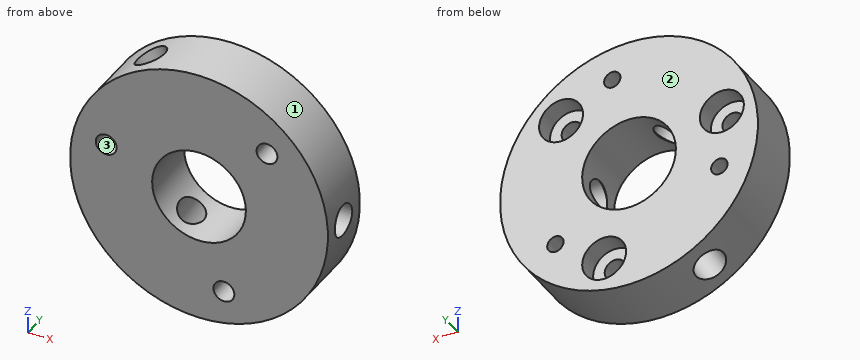
```python
from build123d import *

# Parameters (mm, degrees)
SKETCH1_R                                      = 13.97
BOSS_EXTRUDE1_DEPTH                            = 6.35
CBORE_FOR_2_SOCKET_HEAD_CAP_SCREW1_D           = 2.2606
CBORE_FOR_2_SOCKET_HEAD_CAP_SCREW1_CBORE_D     = 4.7625
CBORE_FOR_2_SOCKET_HEAD_CAP_SCREW1_CBORE_DEPTH = 2.1844
CIRPATTERN1_COUNT                              = 3
CIRPATTERN2_COUNT                              = 3
CIRPATTERN3_COUNT                              = 3
CUT_EXTRUDE2_REACH                             = 22.752
SKETCH16_R                                     = 5.08


with BuildPart() as part:
    # Sketch1 → Boss-Extrude1 (new body)
    with BuildSketch(Plane(origin=(0, 0, 0), x_dir=(1, 0, 0), z_dir=(0, 1, 0))):
        with Locations(Location((0, 0, 0), (0, 0, 270))):
            Circle(SKETCH1_R)
    extrude(amount=BOSS_EXTRUDE1_DEPTH)

    # CBORE for #2 Socket Head Cap Screw1 (through all)
    with Locations(Plane(origin=(0, 6.35, 0), x_dir=(1, 0, 0), z_dir=(0, 1, 0))):
        with Locations((7.363810019, -7.363810019)):
            cbore_for_2_socket_head_cap_screw1 = CounterBoreHole(CBORE_FOR_2_SOCKET_HEAD_CAP_SCREW1_D / 2, CBORE_FOR_2_SOCKET_HEAD_CAP_SCREW1_CBORE_D / 2, CBORE_FOR_2_SOCKET_HEAD_CAP_SCREW1_CBORE_DEPTH)

    # CirPattern1: CBORE for #2 Socket Head Cap Screw1 ×3 about axis
    cirpattern1_axis = Axis((0, 0, 0), (0, 1, 0))
    for i in range(1, CIRPATTERN1_COUNT):
        add(cbore_for_2_socket_head_cap_screw1.rotate(cirpattern1_axis, i * 360 / CIRPATTERN1_COUNT), mode=Mode.SUBTRACT)

    # Sketch10 → Tap Drill for #2-56 Tap2 (revolve, cut)
    with BuildSketch(Plane(origin=(7.977586831, 6.35, -6.693990167), x_dir=(0, 0, 1), z_dir=(1, 0, 0))):
        Polygon((0, 0), (0, 4.59816509), (0.889, 4.064), (0.889, 0), align=None)
    tap_drill_for_2_56_tap2 = revolve(axis=Axis((7.977586831, 12.7, -6.693990167), (0, -1, 0)), mode=Mode.SUBTRACT)

    # CirPattern2: Tap Drill for #2-56 Tap2 ×3 about axis
    cirpattern2_axis = Axis((0, 0, 0), (0, 1, 0))
    for i in range(1, CIRPATTERN2_COUNT):
        add(tap_drill_for_2_56_tap2.rotate(cirpattern2_axis, i * 360 / CIRPATTERN2_COUNT), mode=Mode.SUBTRACT)

    # Sketch15 → Tap Drill for #8-32 Tap2 (revolve, cut)
    with BuildSketch(Plane(origin=(-6.942501454, 3.105629072, 12.122812114), x_dir=(0.8677746681735182, 0, 0.4969578707258195), z_dir=(0, 1, 0))):
        Polygon((0, 0), (0, 10.339292883), (1.7272, 8.89), (1.7272, 0), align=None)
    tap_drill_for_8_32_tap2 = revolve(axis=Axis((-10.098183933, 3.105629072, 17.633181257), (0.4969578707258195, 0, -0.8677746681735182)), mode=Mode.SUBTRACT)

    # CirPattern3: Tap Drill for #8-32 Tap2 ×3 about axis
    cirpattern3_axis = Axis((0, 6.35, 0), (0, -1, 0))
    for i in range(1, CIRPATTERN3_COUNT):
        add(tap_drill_for_8_32_tap2.rotate(cirpattern3_axis, i * 360 / CIRPATTERN3_COUNT), mode=Mode.SUBTRACT)

    # Sketch16 → Cut-Extrude2 (cut, up to next)
    with BuildSketch(Plane(origin=(0, 6.35, 0), x_dir=(1, 0, 0), z_dir=(0, 1, 0)), mode=Mode.PRIVATE) as cut_extrude2_sk1:
        with Locations(Location((0, 0, 0), (0, 0, 270))):
            Circle(SKETCH16_R)
    cut_extrude2_tool1 = extrude(cut_extrude2_sk1.sketch, amount=-CUT_EXTRUDE2_REACH, mode=Mode.PRIVATE) & part.part
    add(cut_extrude2_tool1.solids().sort_by_distance((0, 6.35, 0))[0], mode=Mode.SUBTRACT)


solid = part.part
```
CAD build for the part. Positions are in the model's coordinates, mm. Face numbers are marked on the shaded views. Coordinates: 2 decimals unless noted, no trailing zeros. Write each question's results on one line, items separated by ' | '. Start each with the question number.
Q1. Pull direction Z, two halves, no side cores. Call the marked faces 1, 2 and 3: +Z half, -Z half, draft (parallel to the pull), parting line (faces both ways), or undercut.
Q2. Flat gauge pins, fed straight in: P1, Ø2, axis at y = 1, z = 5, coming from the -X side; P2, Ø1.8, axis at x = -10.06, z = 2.7, coming from the +Y side; P3, Ø2, axis at x = 7.5, y = 3, coming from the -Z side; P4, Ø1.4, axis at x = 8, z = 7.5, coming from the +Y side. Where does each tip first touch, or does it go through?
Q3. Cut at A-A (y = 4.5). Count the separate pieces of the cut face and the enclosed holes in it, then the cut area to 3 significant figures.
Q4. Drill centre lines: probe 1 along Z at (x, y) = (-0.5, 5); probe 2 along Y at (x, z) = (-5.5, 8.5); probe 3 along Y at (x, z) = (4.25, -9). Where is each one in solid material? Low to high. Write a range as from..to.
Found:
1) face 1: parting line | face 2: draft | face 3: undercut
2) P1: x = -13.39 | P2: through | P3: z = -12.37 | P4: y = 4.17
3) separate pieces: 3 | enclosed holes: 6 | area: 417 mm²
4) probe 1: -13.96..-5.06, 5.06..13.96 | probe 2: 0..1.47, 4.74..6.35 | probe 3: 0..4.17
